For this review, take the finished solid that the model builds, in its own axes (mm). A direction names the side the tool comes from. Give positions to 0.01 mm unless a question says otherwise; leave off trailing zeros. Write each loop counter-clockwise with the first axis right and the second up, starting at its lowest first coordinate (ties: lowest second). Pieces come first, ordered by that corner, then holes. Notation, with made-up numbers: (-22, -4) -> (-4, -4) arc R37 cw to (-4, 33) -> close; hole circle Ø7 at (-34, 20.5). An arc over 180 degrees is marked (long way). Return JSON: item names as keys, results as strings.
from build123d import *

# Parameters (mm, degrees)
F1_DEPTH = 20
F2_R     = 40
F5_D     = 8
F5_DEPTH = 10
F5_TIP   = 2.4034424761
F6_D     = 8
F6_DEPTH = 30
F6_TIP   = 2.4034424761


with BuildPart() as f1:
    # F0 (on Right) → F1 (new body)
    with BuildSketch(Plane.YZ):
        Polygon((-177.735026919, 0), (0, 0), (0, 100), (-120, 100), align=None)
        Polygon((-120, 100), (0, 100), (0, 120), (-108.4529946162, 120), align=None)
    extrude(amount=F1_DEPTH)

    # F2
    f2_edges = [f1.edges().sort_by_distance(p)[0] for p in [
        (10, -108.452995, 120),
    ]]
    fillet(f2_edges, radius=F2_R)

    # F5
    with Locations(Plane(origin=(0, 0, 0), x_dir=(0, -1, 0), z_dir=(-1, 0, 0))):
        with Locations((35, 89), (105, 89), (9, 15), (9, 105)):
            Hole(F5_D / 2, depth=F5_DEPTH)
            with Locations((0, 0, -(F5_DEPTH + F5_TIP / 2))):  # 118° drill point
                Cone(0, F5_D / 2, F5_TIP, mode=Mode.SUBTRACT)

    # F6
    with Locations(Plane(origin=(0, 0, 0), x_dir=(1, 0, 0), z_dir=(0, 0, -1))):
        with Locations((11, 120), (11, 50)):
            Hole(F6_D / 2, depth=F6_DEPTH)
            with Locations((0, 0, -(F6_DEPTH + F6_TIP / 2))):  # 118° drill point
                Cone(0, F6_D / 2, F6_TIP, mode=Mode.SUBTRACT)


solid = f1.part
1. Add section C-C, the plane z = 49. State the section outline as (x, y) points, plus the area to 3 significant figures.
Results found:
{"outline": "(0, -149.44) -> (20, -149.44) -> (20, 0) -> (0, 0) -> close", "area": "2,990 mm²"}
2. The part is to be moulded in two halves that separate along Y. For faces 4 (the conical face through (10.849, -119.322, 31.986)), 5 (the conical face through (11.986, -104.449, 88.577)), 6 (the cylindrical face through (10.14, -105.1, 114.79)), 7 (the flat face through (0, -70, 61)), say which applies: +Y half, -Y half, draft (parallel to the pull), parting line (faces both ways), or undercut.
Results found:
{"face 4": "undercut", "face 5": "undercut", "face 6": "-Y half", "face 7": "draft"}
3. For faces 1 (the cylindrical face through (5.07, -105.867, 85.095)), 2 (the flat face through (10, -42, 120)), 3 (the cylindrical face through (11.867, -46.095, 15.21)), list the 3-axis set-ups (+Z, -Z, +X, -X, +Y, -Y) from which the entire face can be reached by the end or side of a thin tool; tool diameter is ignored.
Results found:
{"face 1": "-X", "face 2": "+Z, +X, -X, +Y, -Y", "face 3": "-Z"}
4. Add section D-D, the plane z = 80.5. State the section outline as (x, y) points, plus the area to 3 significant figures.
Results found:
{"outline": "(0, -131.26) -> (20, -131.26) -> (20, 0) -> (0, 0) -> close", "area": "2,630 mm²"}
5. To check wall thickness, follow probe 1 along Z at (x, y) = (3.25, -9); probe 2 along Y at (x, z) = (7, 92); probe 3 along X at (y, z) = (-120, 6). State the ranges of each line that lie inside material, in increasing order.
Results found:
{"probe 1": "z = 0 to 11, 19 to 101, 109 to 120", "probe 2": "y = -124.62 to -107.65, -102.35 to -37.65, -32.35 to 0", "probe 3": "x = 0 to 7, 15 to 20"}
6. Add section A-A, the plane x = 2. State the section outline as (y, z) points, plus the area to 3 significant figures.
Results found:
{"outline": "(-177.74, 0) -> (0, 0) -> (0, 120) -> (-85.36, 120) arc R40 ccw to (-120, 100) -> close; hole circle Ø8 at (-105, 89); hole circle Ø8 at (-35, 89); hole circle Ø8 at (-9, 15); hole circle Ø8 at (-9, 105)", "area": "16,900 mm²"}
7. Add section B-B, the plane z = 25. State the section outline as (x, y) points, plus the area to 3 significant figures.
Results found:
{"outline": "(0, -163.3) -> (20, -163.3) -> (20, 0) -> (0, 0) -> close; hole circle Ø8 at (11, -120); hole circle Ø8 at (11, -50)", "area": "3,170 mm²"}
8. For pin 1 (7 mm diameter, centred on y = -35, z = 89, fed in from -X); pin 2 (5 mm diameter, centred on y = -105, z = 89, fed in from -X); pin 3 (6.5 mm diameter, centred on y = -9, z = 15, fed in from -X), all flat-tipped, find the tip position at first contact; note any pin that passes through.
Results found:
{"pin 1": "stops at x = 10.3", "pin 2": "stops at x = 10.9", "pin 3": "stops at x = 10.45"}
